Source: CAD feature listing. Evaluate the final solid. Frame: model axes, mm. Give positions to 0.01 mm unless a question says otherwise; leave off trailing zeros. Order: outer loops, then holes, each group sorted by start corner. A loop starts at its lowest first (then second) coordinate and runs counter-clockwise, first axis right, second up.
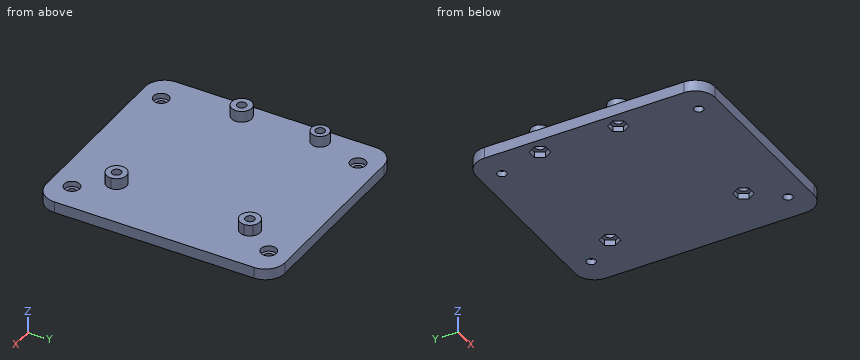
```python
from build123d import *

# Parameters (mm, degrees)
F0_R     = 3.5770918181
F0_R_2   = 3.15
F0_R_3   = 2.75
F0_R_4   = 1.65
F1_DEPTH = 4
F2_DEPTH = 4
F3_DEPTH = 2
F4_R     = 1.65
F5_DEPTH = 2
F6_R     = 7


with BuildPart() as f1:
    # F0 (on Top) → F1 (new body)
    with BuildSketch(Plane.XY):
        with BuildLine():
            Line((17.7415657376, 26.65), (-37.5, 26.65))
            Line((-37.5, 26.65), (-37.5, -26.65))
            Line((-37.5, -26.65), (-34.3, -26.65))
            Line((-34.3, -26.65), (16.5432570596, -26.65))
            ThreePointArc((16.5432570596, -26.65), (17.5844451964, -20.7649139321), (22.5770918181, -24.05))
            ThreePointArc((22.5770918181, -24.05), (22.2850860679, -25.4655548036), (21.4567429404, -26.65))
            Line((21.4567429404, -26.65), (34.3, -26.65))
            Line((34.3, -26.65), (37.5, -26.65))
            Line((37.5, -26.65), (37.5, 26.65))
            Line((37.5, 26.65), (22.8584342624, 26.65))
            ThreePointArc((22.8584342624, 26.65), (23.6126530261, 25.4997836137), (23.8770918181, 24.15))
            ThreePointArc((23.8770918181, 24.15), (18.9502163863, 20.8373469739), (17.7415657376, 26.65))
        make_face()
        with Locations((-31.8, -8.85)):
            Circle(F0_R, mode=Mode.SUBTRACT)
        with Locations((-31.8, 19.05)):
            Circle(F0_R_2, mode=Mode.SUBTRACT)
        with BuildLine():
            Line((-34.3, -26.65), (-37.5, -26.65))
            Line((-37.5, -26.65), (-37.5, -42.5))
            Line((-37.5, -42.5), (37.5, -42.5))
            Line((37.5, -42.5), (37.5, -26.65))
            Line((37.5, -26.65), (34.3, -26.65))
            Line((34.3, -26.65), (21.4567429404, -26.65))
            ThreePointArc((21.4567429404, -26.65), (19, -27.6270918181), (16.5432570596, -26.65))
            Line((16.5432570596, -26.65), (-34.3, -26.65))
        make_face()
        with Locations((-27.5, -35)):
            Circle(F0_R_3, mode=Mode.SUBTRACT)
        with Locations((27.5, -35)):
            Circle(F0_R_3, mode=Mode.SUBTRACT)
        with BuildLine():
            Line((37.5, 42.5), (-37.5, 42.5))
            Line((-37.5, 42.5), (-37.5, 26.65))
            Line((-37.5, 26.65), (17.7415657376, 26.65))
            ThreePointArc((17.7415657376, 26.65), (20.3, 27.7270918181), (22.8584342624, 26.65))
            Line((22.8584342624, 26.65), (37.5, 26.65))
            Line((37.5, 26.65), (37.5, 42.5))
        make_face()
        with Locations((-27.5, 35)):
            Circle(F0_R_3, mode=Mode.SUBTRACT)
        with Locations((27.5, 35)):
            Circle(F0_R_3, mode=Mode.SUBTRACT)
        with Locations((-31.8, -8.85)):
            Circle(F0_R)
        with Locations((-31.8, -8.85)):
            Circle(F0_R_4, mode=Mode.SUBTRACT)
        with BuildLine():
            ThreePointArc((22.5770918181, -24.05), (17.5844451964, -20.7649139321), (16.5432570596, -26.65))
            Line((16.5432570596, -26.65), (21.4567429404, -26.65))
            ThreePointArc((21.4567429404, -26.65), (22.2850860679, -25.4655548036), (22.5770918181, -24.05))
        make_face()
        with Locations((19, -24.05)):
            Circle(F0_R_4, mode=Mode.SUBTRACT)
        with BuildLine():
            Line((22.8584342624, 26.65), (17.7415657376, 26.65))
            ThreePointArc((17.7415657376, 26.65), (18.9502163863, 20.8373469739), (23.8770918181, 24.15))
            ThreePointArc((23.8770918181, 24.15), (23.6126530261, 25.4997836137), (22.8584342624, 26.65))
        make_face()
        with Locations((20.3, 24.15)):
            Circle(F0_R_4, mode=Mode.SUBTRACT)
        with Locations((-31.8, 19.05)):
            Circle(F0_R_2)
        with Locations((-31.8, 19.05)):
            Circle(F0_R_4, mode=Mode.SUBTRACT)
        with Locations((-27.5, 35)):
            Circle(F0_R_3)
        with Locations((-27.5, 35)):
            Circle(F0_R_4, mode=Mode.SUBTRACT)
        with Locations((27.5, 35)):
            Circle(F0_R_3)
        with Locations((27.5, 35)):
            Circle(F0_R_4, mode=Mode.SUBTRACT)
        with Locations((-27.5, -35)):
            Circle(F0_R_3)
        with Locations((-27.5, -35)):
            Circle(F0_R_4, mode=Mode.SUBTRACT)
        with Locations((27.5, -35)):
            Circle(F0_R_3)
        with Locations((27.5, -35)):
            Circle(F0_R_4, mode=Mode.SUBTRACT)
        with BuildLine():
            ThreePointArc((22.8584342624, 26.65), (20.3, 27.7270918181), (17.7415657376, 26.65))
            Line((17.7415657376, 26.65), (22.8584342624, 26.65))
        make_face()
        with BuildLine():
            Line((21.4567429404, -26.65), (16.5432570596, -26.65))
            ThreePointArc((16.5432570596, -26.65), (19, -27.6270918181), (21.4567429404, -26.65))
        make_face()
    extrude(amount=-F1_DEPTH)

    # F0 (on Top) → F2 (join)
    with BuildSketch(Plane.XY):
        with Locations((-31.8, 19.05)):
            Circle(F0_R_2)
        with Locations((-31.8, 19.05)):
            Circle(F0_R_4, mode=Mode.SUBTRACT)
        with Locations((-31.8, -8.85)):
            Circle(F0_R)
        with Locations((-31.8, -8.85)):
            Circle(F0_R_4, mode=Mode.SUBTRACT)
        with BuildLine():
            Line((22.8584342624, 26.65), (17.7415657376, 26.65))
            ThreePointArc((17.7415657376, 26.65), (18.9502163863, 20.8373469739), (23.8770918181, 24.15))
            ThreePointArc((23.8770918181, 24.15), (23.6126530261, 25.4997836137), (22.8584342624, 26.65))
        make_face()
        with Locations((20.3, 24.15)):
            Circle(F0_R_4, mode=Mode.SUBTRACT)
        with BuildLine():
            ThreePointArc((22.8584342624, 26.65), (20.3, 27.7270918181), (17.7415657376, 26.65))
            Line((17.7415657376, 26.65), (22.8584342624, 26.65))
        make_face()
        with BuildLine():
            ThreePointArc((22.5770918181, -24.05), (17.5844451964, -20.7649139321), (16.5432570596, -26.65))
            Line((16.5432570596, -26.65), (21.4567429404, -26.65))
            ThreePointArc((21.4567429404, -26.65), (22.2850860679, -25.4655548036), (22.5770918181, -24.05))
        make_face()
        with Locations((19, -24.05)):
            Circle(F0_R_4, mode=Mode.SUBTRACT)
        with BuildLine():
            Line((21.4567429404, -26.65), (16.5432570596, -26.65))
            ThreePointArc((16.5432570596, -26.65), (19, -27.6270918181), (21.4567429404, -26.65))
        make_face()
    extrude(amount=F2_DEPTH)

    # F0 (on Top) → F3 (cut)
    with BuildSketch(Plane.XY):
        with Locations((-27.5, 35)):
            Circle(F0_R_3)
        with Locations((-27.5, 35)):
            Circle(F0_R_4, mode=Mode.SUBTRACT)
        with Locations((27.5, 35)):
            Circle(F0_R_3)
        with Locations((27.5, 35)):
            Circle(F0_R_4, mode=Mode.SUBTRACT)
        with Locations((-27.5, -35)):
            Circle(F0_R_3)
        with Locations((-27.5, -35)):
            Circle(F0_R_4, mode=Mode.SUBTRACT)
        with Locations((27.5, -35)):
            Circle(F0_R_3)
        with Locations((27.5, -35)):
            Circle(F0_R_4, mode=Mode.SUBTRACT)
    extrude(amount=-F3_DEPTH, mode=Mode.SUBTRACT)

    # F4 (on face) → F5 (cut)
    with BuildSketch(Plane(origin=(0, 0, -4), x_dir=(1, 0, 0), z_dir=(0, 0, -1))):
        Polygon((18.6256842194, -27.05), (21.9743157806, -27.05), (23.6486315613, -24.15), (21.9743157806, -21.25), (18.6256842194, -21.25), (16.9513684387, -24.15), align=None)
        with Locations((20.3, -24.15)):
            Circle(F4_R, mode=Mode.SUBTRACT)
        Polygon((-33.4743157806, -21.95), (-30.1256842194, -21.95), (-28.4513684387, -19.05), (-30.1256842194, -16.15), (-33.4743157806, -16.15), (-35.1486315613, -19.05), align=None)
        with Locations((-31.8, -19.05)):
            Circle(F4_R, mode=Mode.SUBTRACT)
        Polygon((17.3256842194, 21.15), (20.6743157806, 21.15), (22.3486315613, 24.05), (20.6743157806, 26.95), (17.3256842194, 26.95), (15.6513684387, 24.05), align=None)
        with Locations((19, 24.05)):
            Circle(F4_R, mode=Mode.SUBTRACT)
        Polygon((-33.4743157806, 5.95), (-30.1256842194, 5.95), (-28.4513684387, 8.85), (-30.1256842194, 11.75), (-33.4743157806, 11.75), (-35.1486315613, 8.85), align=None)
        with Locations((-31.8, 8.85)):
            Circle(F4_R, mode=Mode.SUBTRACT)
    extrude(amount=-F5_DEPTH, mode=Mode.SUBTRACT)

    # F6
    f6_edges = [f1.edges().sort_by_distance(p)[0] for p in [
        (-37.5, 42.5, -2),
        (-37.5, -42.5, -2),
        (37.5, -42.5, -2),
        (37.5, 42.5, -2),
    ]]
    fillet(f6_edges, radius=F6_R)


solid = f1.part
```
1) Section query A-A, the plane z = 3. Return the cut outline in (x, y).
Report:
outline: circle Ø7.15 at (-31.8, -8.85); circle Ø6.3 at (-31.8, 19.05); circle Ø7.15 at (19, -24.05); circle Ø7.15 at (20.3, 24.15); hole circle Ø3.3 at (-31.8, -8.85); hole circle Ø3.3 at (-31.8, 19.05); hole circle Ø3.3 at (19, -24.05); hole circle Ø3.3 at (20.3, 24.15)
2) Material intervals for L1, parallel to Y at x = -27.5, z = -2.9; L2, parallel to Y at x = -27.5, z = -0.85; L3, parallel to Y at x = 20.3, z = 2.15, sorted ascending.
Report:
L1: y = -42.5 to -36.65, -33.35 to 33.35, 36.65 to 42.5
L2: y = -42.5 to -37.75, -32.25 to 32.25, 37.75 to 42.5
L3: y = -27.38 to -25.07, -23.03 to -20.72, 20.57 to 22.5, 25.8 to 27.73
3) Section query C-C, the plane x = 14. Return the cut outline in (y, z), and give its area (3 significant figures).
Report:
outline: (-42.5, -4) - (42.5, -4) - (42.5, 0) - (-42.5, 0) - close
area: 340 mm2
4) Section query B-B, the plane x = -31.8. Return the cut outline in (y, z), and give its area (3 significant figures).
Report:
outline: (-42.38, -4) - (-11.75, -4) - (-11.75, -2) - (-10.5, -2) - (-10.5, 4) - (-12.43, 4) - (-12.43, 0) - (-42.38, 0) - close; (-7.2, -2) - (-5.95, -2) - (-5.95, -4) - (16.15, -4) - (16.15, -2) - (17.4, -2) - (17.4, 4) - (15.9, 4) - (15.9, 0) - (-5.27, 0) - (-5.27, 4) - (-7.2, 4) - close; (20.7, -2) - (21.95, -2) - (21.95, -4) - (42.38, -4) - (42.38, 0) - (22.2, 0) - (22.2, 4) - (20.7, 4) - close
area: 330 mm2
5) Pin query (flat end, axial travel): pin 1 (9 mm diameter, centred on x = 27.5, y = 35, fed in from +Z); pin 2 (2 mm diameter, centred on y = 17.5, z = 2, fed in from -X); pin 3 (1.5 mm diameter, centred on y = 6.5, z = 0.5, fed in from -X); pin 4 (4 mm diameter, centred on x = 20.3, y = 24.15, fed in from -Z). Return the tip coordinate at first contact, or that it passes through.
Report:
pin 1: stops at z = 0
pin 2: stops at x = -34.9
pin 3: stops at x = -37.5
pin 4: stops at z = -2
